```python
from build123d import *

# Parameters (mm, degrees)
F0_R     = 6
F0_R_2   = 4
F1_DEPTH = 3
F2_DEPTH = 37
F3_DEPTH = 34
F4_DEPTH = 1
F5_DEPTH = 5000
F6_R     = 10
F7_R     = 1


with BuildPart() as f1:
    # F0 (on Top) → F1 (new body)
    with BuildSketch(Plane.XY):
        Polygon((0, 14.1421356237), (-45.7365440327, 59.8786796564), (-59.8786796564, 45.7365440327), (0, -14.1421356237), (59.8786796564, 45.7365440327), (45.7365440327, 59.8786796564), align=None)
        Circle(F0_R, mode=Mode.SUBTRACT)
        Polygon((-45.7365440327, 59.8786796564), (-52.8076118446, 66.9497474683), (-66.9497474683, 52.8076118446), (-59.8786796564, 45.7365440327), align=None)
        Polygon((52.8076118446, 66.9497474683), (45.7365440327, 59.8786796564), (59.8786796564, 45.7365440327), (66.9497474683, 52.8076118446), align=None)
        Circle(F0_R)
        Circle(F0_R_2, mode=Mode.SUBTRACT)
        Polygon((-52.8076118446, 66.9497474683), (-54.9289321881, 69.0710678119), (-69.0710678119, 54.9289321881), (-66.9497474683, 52.8076118446), align=None)
        Polygon((54.9289321881, 69.0710678119), (52.8076118446, 66.9497474683), (66.9497474683, 52.8076118446), (69.0710678119, 54.9289321881), align=None)
        Circle(F0_R_2)
    extrude(amount=F1_DEPTH)

    # F0 (on Top) → F2 (join)
    with BuildSketch(Plane.XY):
        Polygon((-52.8076118446, 66.9497474683), (-54.9289321881, 69.0710678119), (-69.0710678119, 54.9289321881), (-66.9497474683, 52.8076118446), align=None)
        Polygon((-45.7365440327, 59.8786796564), (-52.8076118446, 66.9497474683), (-66.9497474683, 52.8076118446), (-59.8786796564, 45.7365440327), align=None)
        Polygon((52.8076118446, 66.9497474683), (45.7365440327, 59.8786796564), (59.8786796564, 45.7365440327), (66.9497474683, 52.8076118446), align=None)
        Polygon((54.9289321881, 69.0710678119), (52.8076118446, 66.9497474683), (66.9497474683, 52.8076118446), (69.0710678119, 54.9289321881), align=None)
    extrude(amount=-F2_DEPTH)

    # F0 (on Top) → F3 (cut)
    with BuildSketch(Plane.XY):
        Polygon((-45.7365440327, 59.8786796564), (-52.8076118446, 66.9497474683), (-66.9497474683, 52.8076118446), (-59.8786796564, 45.7365440327), align=None)
        Polygon((52.8076118446, 66.9497474683), (45.7365440327, 59.8786796564), (59.8786796564, 45.7365440327), (66.9497474683, 52.8076118446), align=None)
    extrude(amount=-F3_DEPTH, mode=Mode.SUBTRACT)

    # F0 (on Top) → F4 (cut)
    with BuildSketch(Plane.XY):
        Circle(F0_R)
        Circle(F0_R_2, mode=Mode.SUBTRACT)
    extrude(amount=F4_DEPTH, mode=Mode.SUBTRACT)

    # F0 (on Top) → F5 (cut)
    with BuildSketch(Plane.XY):
        Circle(F0_R_2)
    extrude(amount=F5_DEPTH, mode=Mode.SUBTRACT)

    # F6
    f6_edges = [f1.edges().sort_by_distance(p)[0] for p in [
        (0, -14.142136, 1.5),
        (0, 14.142136, 1.5),
    ]]
    fillet(f6_edges, radius=F6_R)

    # F7
    f7_edges = [f1.edges().sort_by_distance(p)[0] for p in [
        (62, 62, 3),
        (59.87868, 59.87868, 0),
        (62, 62, -37),
        (59.87868, 59.87868, -34),
        (-62, 62, -37),
        (-62, 62, 3),
        (-59.87868, 59.87868, 0),
        (-59.87868, 59.87868, -34),
    ]]
    fillet(f7_edges, radius=F7_R)


solid = f1.part
```
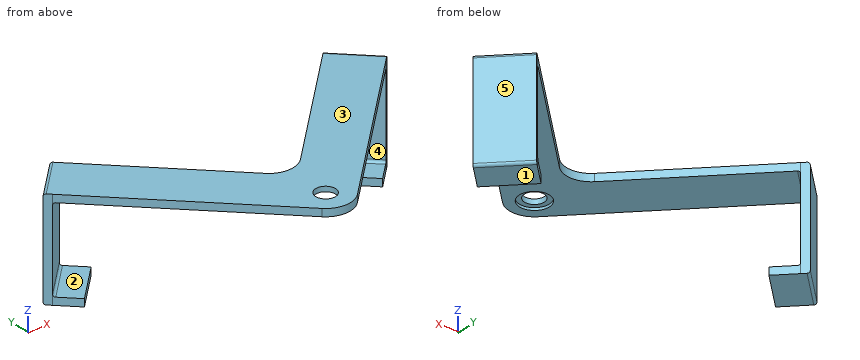
Check sheet for the modelled part. Datum: model origin and axes. Units: mm. Face numbers are marked on the shaded views. A direction names the side the tool comes from. Round coordinates to 2 decimals unless told otherwise and drop trailing zeros. Order: outer loops, then holes, each group sorted by start corner. A loop starts at its lowest first (then second) coordinate and runs counter-clockwise, first axis right, second up.
1) Section check A-A (x = 0). Record the boundary of the cut face in (y, z).
2) Section check B-B (z = -19). Record the boundary of the cut face in (x, y).
3) Mould release check, pull along Z, two halves, no side actions. Record for the marked faces 1, 2 and 3: +Z half, -Z half, draft (parallel to the pull), parting line (faces both ways), or undercut.
4) Go/stop test with a flat-tipped pin: pin 1 Ø1 at (x, y) = (16, 12) entering from -Z. Record where the tip stops, or that it passes through.
5) Section check D-D (y = 38). Record the boundary of the cut face in (x, z).
6) Scan lines: line 1 (Y direction, x = 0, z = 0.7); line 2 (Z direction, x = 9, y = 12.5); line 3 (Y direction, x = 0, z = 1.95). Record each from-to range of solid material in increasing order.
7) Section check C-C (y = 0). Record the boundary of the cut face in (x, z).
8) Tool access check on the marked faces 4 and 5. Record the directions out of +Z, -Z, +X, -X, +Y, -Y that give a thin tool (end or side, any length) a straight path to the whole face; none if there is none.
Result:
1. outline: (-10, 0) - (-6, 0) - (-6, 1) - (-4, 1) - (-4, 3) - (-10, 3) - close; (4, 1) - (6, 1) - (6, 0) - (18.28, 0) - (18.28, 3) - (4, 3) - close
2. outline: (-69.07, 54.93) - (-66.95, 52.81) - (-52.81, 66.95) - (-54.93, 69.07) - close; (52.81, 66.95) - (66.95, 52.81) - (69.07, 54.93) - (54.93, 69.07) - close
3. face 1: -Z half
3. face 2: undercut
3. face 3: +Z half
4. pin 1: stops at z = 0
5. outline: (-52.14, 0) - (-23.86, 0) - (-23.86, 3) - (-52.14, 3) - close; (23.86, 0) - (52.14, 0) - (52.14, 3) - (23.86, 3) - close
6. line 1: y = -10 to -6, 6 to 18.28
6. line 2: z = 0 to 3
6. line 3: y = -10 to -4, 4 to 18.28
7. outline: (-14.14, 0) - (-6, 0) - (-6, 1) - (-4, 1) - (-4, 3) - (-14.14, 3) - close; (4, 1) - (6, 1) - (6, 0) - (14.14, 0) - (14.14, 3) - (4, 3) - close
8. face 4: -Y
8. face 5: +Z, -Z, +X, +Y
